Design review of the part built by this model. Coordinates are the model's own, in mm. Face numbers are marked on the shaded views. A direction names the side the tool comes from. Coordinates: 2 decimals unless noted, no trailing zeros. Loops run counter-clockwise (first coordinate to the right, second up) from the corner with the lowest first, then second, coordinate; pieces in that order, holes last. Notation, with made-up numbers: M 72,-16.5 L 119,-16.5 A18 cw 119,-4.5 Z; hole C 34.5,-14.5 d2. An arc over 180 degrees is marked long. One line per item, written item: value.
```python
from build123d import *

# Parameters (mm, degrees)
SKETCH1_W           = 50
SKETCH1_H           = 30
SKETCH1_R           = 3.75
BOSS_EXTRUDE1_DEPTH = 2.5
BOSS_EXTRUDE2_START = -20
SKETCH3_R           = 2.5
BOSS_EXTRUDE2_DEPTH = 10
LPATTERN1_COUNT     = 2
LPATTERN1_PITCH     = 20
SKETCH5_R           = 1.575
CUT_EXTRUDE1_DEPTH  = 50
SKETCH6_R           = 2.5
CUT_EXTRUDE2_DEPTH  = 10
LPATTERN2_COUNT     = 3
LPATTERN2_PITCH     = 20
ESCALA1_SCALE       = 0.5


with BuildPart() as part:
    # Sketch1 → Boss-Extrude1 (new body)
    with BuildSketch(Plane(origin=(0, 0, 0), x_dir=(0, 0, -1), z_dir=(1, 0, 0))):
        with Locations((25, 15)):
            Rectangle(SKETCH1_W, SKETCH1_H)
        with Locations((40, 20)):
            Circle(SKETCH1_R, mode=Mode.SUBTRACT)
        with Locations((25, 10)):
            Circle(SKETCH1_R, mode=Mode.SUBTRACT)
        with Locations((10, 20)):
            Circle(SKETCH1_R, mode=Mode.SUBTRACT)
    extrude(amount=BOSS_EXTRUDE1_DEPTH)

    # Sketch3 → Boss-Extrude2 (add)
    with BuildSketch(Plane(origin=(0, 0, -50), x_dir=(-1, 0, 0), z_dir=(0, 0, -1)).offset(BOSS_EXTRUDE2_START)):
        with Locations((-2.5, 30)):
            Circle(SKETCH3_R)
    boss_extrude2 = extrude(amount=BOSS_EXTRUDE2_DEPTH)

    # LPattern1: Boss-Extrude2 ×2
    with Locations(*[(0, 0, i * LPATTERN1_PITCH) for i in range(1, LPATTERN1_COUNT)]):
        add(boss_extrude2)

    # Sketch5 → Cut-Extrude1 (cut)
    with BuildSketch(Plane(origin=(0, 0, -50), x_dir=(-1, 0, 0), z_dir=(0, 0, -1))):
        with Locations((-2.5, 30)):
            Circle(SKETCH5_R)
    extrude(amount=-CUT_EXTRUDE1_DEPTH, mode=Mode.SUBTRACT)

    # Sketch6 → Cut-Extrude2 (cut)
    with BuildSketch(Plane(origin=(0, 0, -50), x_dir=(-1, 0, 0), z_dir=(0, 0, -1))):
        with Locations((-2.5, 30)):
            Circle(SKETCH6_R)
    cut_extrude2 = extrude(amount=-CUT_EXTRUDE2_DEPTH, mode=Mode.SUBTRACT)

    # LPattern2: Cut-Extrude2 ×3
    with Locations(*[(0, 0, i * LPATTERN2_PITCH) for i in range(1, LPATTERN2_COUNT)]):
        add(cut_extrude2, mode=Mode.SUBTRACT)


with BuildPart() as part_1:
    # Escala1: scaled about (0, 0, 0)
    add(part.part.scale(ESCALA1_SCALE))


solid = part_1.part
```
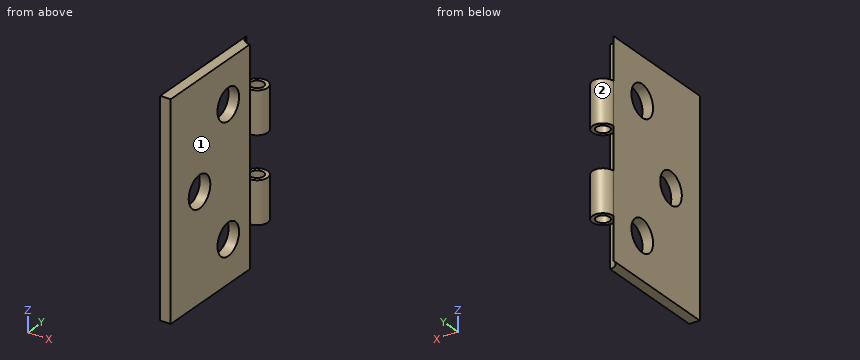
(1) We need section C-C on z = -12.5. State the section outline as (x, y) points (3 decimals).
Reply:
outline: M 0,0 L 1.25,0 L 1.25,3.125 L 0,3.125 Z; M 0,6.875 L 1.25,6.875 L 1.25,13.75 A1.25 cw 0,15 Z
(2) To check wall thickness, follow line 1 along X through (y, z) = (15, -7.45); line 2 along Z through (x, y) = (0.8, 11.25); line 3 along Y through (x, z) = (0.55, -19.5). State the ranges of each line that lie inside material, in increasing order. Write a range as [from, to].
Reply:
line 1: x = [0, 0.46], [2.04, 2.5]
line 2: z = [-25, -21.4], [-18.6, -6.4], [-3.6, 0]
line 3: y = [0, 8.19], [11.81, 14.64], [15.36, 16.04]
(3) Tool access review of the marked faces 1 and 2: name each direction out of +Z, -Z, +X, -X, +Y, -Y from which nothing blocks a thin tool from reaching the whole face with its end or side.
Reply:
face 1: +Z, -Z, +X, -Y
face 2: +Z, -Z
(4) Insertion check: pin 1 (1.5 mm diameter, centred on x = 1.5, y = 5.5, fed in from -Z); pin 2 (1.5 mm diameter, centred on y = 4, z = -18.5, fed in from +X); pin 3 (1.2 mm diameter, centred on x = 1.5, y = 15, fed in from +Z); pin 4 (0.8 mm diameter, centred on x = 1, y = 15.5, fed in from -Z). Each pin has a flat end and moves straight along its axis. Give the tip position at first contact, or say it passes through.
Reply:
pin 1: stops at z = -25
pin 2: stops at x = 1.25
pin 3: stops at z = -5
pin 4: stops at z = -20
(5) We need section D-D on y = 8.75. State the section outline as (x, z) points.
Reply:
outline: M 0,-25 L 1.25,-25 L 1.25,-21.4 L 0,-21.4 Z; M 0,-18.6 L 1.25,-18.6 L 1.25,-6.4 L 0,-6.4 Z; M 0,-3.6 L 1.25,-3.6 L 1.25,0 L 0,0 Z
(6) We need section B-B on y = 5. State the section outline as (x, z) points (3 decimals).
Reply:
outline: M 0,-25 L 1.25,-25 L 1.25,-14.375 L 0,-14.375 Z; M 0,-10.625 L 1.25,-10.625 L 1.25,0 L 0,0 Z
(7) We need section A-A on x = 0.95. State the section outline as (y, z) points (3 decimals).
Reply:
outline: M 0,-25 L 13.787,-25 L 13.787,-20 L 14.272,-20 L 14.272,-15 L 13.787,-15 L 13.787,-10 L 14.272,-10 L 14.272,-5 L 13.787,-5 L 13.787,0 L 0,0 Z; M 15.728,-20 L 16.213,-20 L 16.213,-15 L 15.728,-15 Z; M 15.728,-10 L 16.213,-10 L 16.213,-5 L 15.728,-5 Z; hole C 5,-12.5 d3.75; hole C 10,-20 d3.75; hole C 10,-5 d3.75
